from build123d import *

# Parameters (mm, degrees)
F0_W          = 8
F0_H          = 10
F1_DEPTH      = 8
F2_SIZE       = 4
F4_DEPTH      = 4
F5_DEPTH      = 3
F6_R          = 3.3
F7_DEPTH      = 3
F9_DEPTH      = 1.4
F11_R         = 1.7
F12_DEPTH     = 4
F13_R         = 2
F14_DEPTH     = 12.5
F15_T1_DEPTH  = 13.1433659759
F15_T6_DEPTH  = 13.1433659759
F15_S7_R      = 3
F15_T8_DEPTH  = 8
F16_W         = 1.5
F16_H         = 1.0667801354
F16_H_2       = 8
F16_H_3       = 0.8089432385
F17_DEPTH     = 1
F18_T4_DEPTH  = 11.5268513298
F18_S7_R      = 3.3
F18_T8_DEPTH  = 7
F18_T12_DEPTH = 11.5268513298
F18_S14_R     = 3.3
F18_T15_DEPTH = 7
F19_R         = 0.75
F20_DEPTH     = 25


# Not quite as in the source:
# - a fillet or chamfer that OpenCascade refuses, or shapes differently, is made with other operations: its cross-section is extruded or revolved along the edge and cut away or added


with BuildPart() as f1:
    # F0 (on Top) → F1 (new body)
    with BuildSketch(Plane.XY):
        with Locations((0, 5)):
            Rectangle(F0_W, F0_H)
    extrude(amount=F1_DEPTH)

    # F2
    f2_edges = [f1.edges().sort_by_distance(p)[0] for p in [
        (0, 0, 8),
        (0, 10, 8),
    ]]
    chamfer(f2_edges, length=F2_SIZE)

    # F3 (on Right) → F4 (join, symmetric)
    with BuildSketch(Plane.YZ):
        with BuildLine():
            ThreePointArc((2.1213203436, 6.1213203436), (-2.7716385975, 5.1480502971), (0, 1))
            Line((0, 1), (0, 4))
            Line((0, 4), (2.1213203436, 6.1213203436))
        make_face()
    extrude(amount=F4_DEPTH, both=True)

    # F3 (on Right) → F5 (join, symmetric)
    with BuildSketch(Plane.YZ):
        with BuildLine():
            Line((10, 4), (10, 1))
            ThreePointArc((10, 1), (12.1213203436, 1.8786796564), (13, 4))
            ThreePointArc((13, 4), (11.1480502971, 6.7716385975), (7.8786796564, 6.1213203436))
            Line((7.8786796564, 6.1213203436), (10, 4))
        make_face()
    extrude(amount=F5_DEPTH, both=True)

    # F6 (on Right) → F7 (cut, symmetric)
    with BuildSketch(Plane.YZ):
        with Locations((0, 4.1532493821)):
            Circle(F6_R)
    extrude(amount=F7_DEPTH, both=True, mode=Mode.SUBTRACT)

    # F8 (on face) → F9 (cut)
    with BuildSketch(Plane(origin=(-4, 0, 0), x_dir=(0, -1, 0), z_dir=(-1, 0, 0))):
        with BuildLine():
            Line((-10, 4), (-7.7019029611, 6.2980970389))
            ThreePointArc((-7.7019029611, 6.2980970389), (-13.0026084807, 5.2437211552), (-10, 0.75))
            Line((-10, 0.75), (-10, 4))
        make_face()
        with BuildLine():
            ThreePointArc((-10, 0.75), (-7.7019029611, 1.7019029611), (-6.75, 4))
            ThreePointArc((-6.75, 4), (-6.9973915193, 5.2437211552), (-7.7019029611, 6.2980970389))
            Line((-7.7019029611, 6.2980970389), (-10, 4))
            Line((-10, 4), (-10, 0.75))
        make_face()
    extrude(amount=-F9_DEPTH, mode=Mode.SUBTRACT)

    # F10: F1 across plane


with BuildPart() as f1_1:
    add(f1.part)
    add(f1.part.mirror(Plane.YZ), mode=Mode.INTERSECT)

    # F11 (on Right) → F12 (join, symmetric)
    with BuildSketch(Plane.YZ):
        with Locations((10, 4)):
            Circle(F11_R)
    extrude(amount=F12_DEPTH, both=True)

    # F13 (on Right) → F14 (cut, symmetric)
    with BuildSketch(Plane.YZ):
        with Locations((0, 4)):
            Circle(F13_R)
    extrude(amount=F14_DEPTH, both=True, mode=Mode.SUBTRACT)

    # F15: chamfer of 1 on 2 edges, made by hand

    # F15_s2 → F15_t1 (cut)
    with BuildSketch(Plane.YZ.offset(-6.571682988)):
        Polygon((1, 0), (0, 1), (0, 0), align=None)
    extrude(amount=F15_T1_DEPTH, mode=Mode.SUBTRACT)


with BuildPart() as f15_tool4:
    # F15_s5 → F15_t6 (new body)
    with BuildSketch(Plane.YZ.offset(6.571682988)):
        Polygon((9, 0), (10, 1), (10, 0), align=None)
    extrude(amount=-F15_T6_DEPTH)

    # F15_s7 → F15_t8 (cut, symmetric)
    with BuildSketch(Plane.YZ):
        with Locations((10, 4)):
            Circle(F15_S7_R)
    extrude(amount=F15_T8_DEPTH, both=True, mode=Mode.SUBTRACT)


with BuildPart() as f1_2:
    add(f1_1.part)

    # F15_t3: cut F15_tool4
    add(f15_tool4.part, mode=Mode.SUBTRACT)

    # F16 (on face) → F17 (cut)
    with BuildSketch(Plane(origin=(0, 0, 0), x_dir=(1, 0, 0), z_dir=(0, 0, -1))):
        with Locations((0, -9.5333900677)):
            Rectangle(F16_W, F16_H)
        with Locations((0, -5)):
            Rectangle(F16_W, F16_H_2)
        with Locations((0, -0.5955283808)):
            Rectangle(F16_W, F16_H_3)
    extrude(amount=-F17_DEPTH, mode=Mode.SUBTRACT)

    # F18: fillet of radius 0.5 on 2 edges, made by hand


with BuildPart() as f18_tool2:
    # F18_s3 → F18_t4 (new body)
    with BuildSketch(Plane.XZ.offset(0.2768513298)):
        with BuildLine():
            ThreePointArc((-0.75, 0.5), (-0.6035533906, 0.8535533906), (-0.25, 1))
            Line((-0.25, 1), (-0.75, 1))
            Line((-0.75, 1), (-0.75, 0.5))
        make_face()
    extrude(amount=-F18_T4_DEPTH)

    split(bisect_by=Plane(origin=(0, 0.5, 0.5), x_dir=(1, 0, 0), z_dir=(0, 0.7071067812, 0.7071067812)), keep=Keep.TOP)

    split(bisect_by=Plane(origin=(0, 4.5, -4.5), x_dir=(1, 0, 0), z_dir=(0, -0.7071067812, 0.7071067812)), keep=Keep.TOP)

    # F18_s7 → F18_t8 (cut, symmetric)
    with BuildSketch(Plane.YZ.offset(-0.5)):
        with Locations((0, 4.1532493821)):
            Circle(F18_S7_R)
    extrude(amount=F18_T8_DEPTH, both=True, mode=Mode.SUBTRACT)


with BuildPart() as f1_3:
    add(f1_2.part)

    # F18_t1: union F18_tool2
    add(f18_tool2.part)


with BuildPart() as f18_tool10:
    # F18_s11 → F18_t12 (new body)
    with BuildSketch(Plane.XZ.offset(-11.25)):
        with BuildLine():
            ThreePointArc((0.75, 0.5), (0.6035533906, 0.8535533906), (0.25, 1))
            Line((0.25, 1), (0.75, 1))
            Line((0.75, 1), (0.75, 0.5))
        make_face()
    extrude(amount=F18_T12_DEPTH)

    split(bisect_by=Plane(origin=(0, 0.5, 0.5), x_dir=(1, 0, 0), z_dir=(0, 0.7071067812, 0.7071067812)), keep=Keep.TOP)

    # F18_s14 → F18_t15 (cut, symmetric)
    with BuildSketch(Plane.YZ.offset(0.5)):
        with Locations((0, 4.1532493821)):
            Circle(F18_S14_R)
    extrude(amount=F18_T15_DEPTH, both=True, mode=Mode.SUBTRACT)

    split(bisect_by=Plane(origin=(0, 4.5, -4.5), x_dir=(1, 0, 0), z_dir=(0, -0.7071067812, 0.7071067812)), keep=Keep.TOP)


with BuildPart() as f1_4:
    add(f1_3.part)

    # F18_t9: union F18_tool10
    add(f18_tool10.part)

    # F19 (on Front) → F20 (cut)
    with BuildSketch(Plane.XZ):
        with Locations((0, 6.8)):
            Circle(F19_R)
    extrude(amount=-F20_DEPTH, mode=Mode.SUBTRACT)


solid = f1_4.part
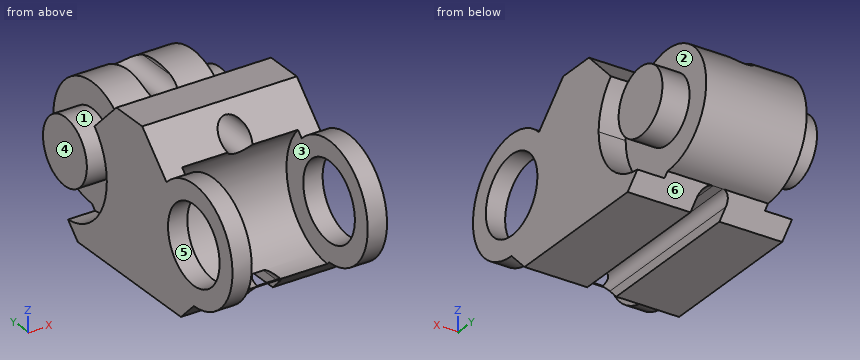
Source: CAD feature listing. Evaluate the final solid. Frame: model axes, mm. Face numbers are marked on the shaded views. A direction names the side the tool comes from. Give positions to 0.01 mm unless a question says otherwise; leave off trailing zeros. Write each loop counter-clockwise with the first axis right and the second up, starting at its lowest first coordinate (ties: lowest second). Pieces come first, ordered by that corner, then holes. Notation, with made-up numbers: (-17.75, 38.5) -> (11.25, 38.5) arc R24 ccw to (11.25, 75.5) -> close; hole circle Ø8 at (78, 18.5). An arc over 180 degrees is marked (long way). Return JSON: item names as keys, results as strings. Group by question number.
1. Section B-B, the plane x = 1.25. Output: boundary loops of the cut face in (y, z).
2. Material intervals for line 1 (X direction, y = 10, z = 6.8); line 2 (Z direction, x = 0, y = 5.25); line 3 (X direction, y = 6.75, z = 6.8), sorted ascending. Write a range as from..to.
3. Mould query, pull axis Y, two halves, no side actions, for the marked faces 4, 5 and 6. Classes: +Y half, -Y half, draft (parallel to the pull), parting line (faces both ways), or undercut.
4. Section A-A, the plane z = 4.25. Output: boundary loops of the cut face in (x, y), then the cut area to 3 significant figures.
5. Pin query (flat end, axial travel): pin 1 Ø1 at (x, y) = (-0.5, 2) entering from +Z; pin 2 Ø2.5 at (x, z) = (0, 6.8) entering from -Y; pin 3 Ø3.5 at (y, z) = (0, 4) entering from -X. Return the tip coordinate at first contact, or that it passes through.
6. Section C-C, the plane y = 7. Output: boundary loops of the cut face in (x, z), then the cut area to 3 significant figures.
7. Access query for the marked faces 1, 2 and 3. Directions: +Z, -Z, +X, -X, +Y, -Y. A direction counts if a zero-diameter tool reaches every point of the face in a straight line with its end or side. Return the directions, or none.
Determined:
{
 "1": {"outline": "(0.14, 0.86) -> (1, 0) -> (9, 0) -> (10, 1) arc R3 ccw (long way) to (7.88, 6.12) -> (6, 8) -> (4, 8) -> (2.41, 6.41) arc R3.3 cw to start"},
 "2": {"line 1": "x = -2.6..-0.75, 0.75..2.6", "line 2": "z = 1..6.05, 7.55..8", "line 3": "x = -4..-0.75, 0.75..4"},
 "3": {"face 4": "draft", "face 5": "undercut", "face 6": "+Y half"},
 "4": {"outline": "(-4, -2.99) -> (-3, -2.99) -> (-3, -1.98) -> (-4, -1.98) -> close; (-4, 1.98) -> (-3, 1.98) -> (-3, 3.3) -> (3, 3.3) -> (3, 1.98) -> (4, 1.98) -> (4, 6.76) -> (2.6, 6.76) -> (2.6, 8.32) -> (4, 8.32) -> (4, 11.68) -> (2.6, 11.68) -> (2.6, 12.99) -> (-2.6, 12.99) -> (-2.6, 11.68) -> (-4, 11.68) -> (-4, 8.32) -> (-2.6, 8.32) -> (-2.6, 6.76) -> (-4, 6.76) -> close; (3, -2.99) -> (4, -2.99) -> (4, -1.98) -> (3, -1.98) -> close", "area": "74.1 mm2"},
 "5": {"pin 1": "stops at z = 6.47", "pin 2": "stops at y = 2.41", "pin 3": "passes through"},
 "6": {"outline": "(-4, 0) -> (-0.75, 0) -> (-0.75, 0.5) arc R0.5 cw to (-0.25, 1) -> (0.25, 1) arc R0.5 cw to (0.75, 0.5) -> (0.75, 0) -> (4, 0) -> (4, 2.75) -> (2.6, 2.75) -> (2.6, 5.25) -> (4, 5.25) -> (4, 7) -> (0.72, 7) arc R0.75 cw (long way) to (-0.72, 7) -> (-4, 7) -> (-4, 5.25) -> (-2.6, 5.25) -> (-2.6, 2.75) -> (-4, 2.75) -> close", "area": "46.4 mm2"},
 "7": {"face 1": "-X", "face 2": "+X", "face 3": "-Y"}
}
